```python
from build123d import *

# Parameters (mm, degrees)
SKETCH_1_W           = 20
SKETCH_1_H           = 39.9
SKETCH_1_R           = 1.5
EXTRUDE_1_DEPTH      = 5
EXTRUDE_1_2_DEPTH    = 5
EXTRUDE_2_DEPTH      = 4
EXTRUDE_2_DEPTH_BACK = 4
FILLET_1_R           = 14
SKETCH_3_R           = 1.5
CUT_EXTRUDE_1_DEPTH  = 11
FILLET_2_R           = 5
SKETCH_4_W           = 4
SKETCH_4_H           = 12
EXTRUDE_3_DEPTH      = 7
CUT_EXTRUDE_2_DEPTH  = 148
EXTRUDE_4_DEPTH      = 4
EXTRUDE_4_DEPTH_BACK = 8
SKETCH_6_W           = 4
SKETCH_6_H           = 30.5
SKETCH_10_W          = 20
SKETCH_10_H          = 6
SKETCH_10_H_2        = 5
EXTRUDE_6_DEPTH      = 4
CUT_EXTRUDE_5_DEPTH  = 6
SKETCH_13_R          = 1.5
CUT_EXTRUDE_6_DEPTH  = 6
EXTRUDE_8_DEPTH      = 4
SKETCH_19_W          = 8
SKETCH_19_H          = 15
SKETCH_19_R          = 1.5
SKETCH_19_H_2        = 8
EXTRUDE_9_DEPTH      = 5
CHAMFER_START        = -4
CHAMFER_1_DEPTH      = 8
FILLET_13_R          = 1
FILLET_14_R          = 10
FILLET_15_R          = 3


with BuildPart() as part:
    # Sketch 1 → Extrude 1 (new body)
    with BuildSketch(Plane.XY):
        with Locations((45, 0)):
            Rectangle(SKETCH_1_W, SKETCH_1_H)
        with Locations((37.5, 8)):
            Circle(SKETCH_1_R, mode=Mode.SUBTRACT)
        with Locations(Location((52.5, 8, 0), (0, 0, 180))):
            Circle(SKETCH_1_R, mode=Mode.SUBTRACT)
        with Locations((52.5, -8)):
            Circle(SKETCH_1_R, mode=Mode.SUBTRACT)
        with Locations(Location((37.5, -8, 0), (0, 0, 180))):
            Circle(SKETCH_1_R, mode=Mode.SUBTRACT)
    extrude(amount=EXTRUDE_1_DEPTH)



with BuildPart() as body_2:
    # Sketch 1 → Extrude 1 2 (new body)
    with BuildSketch(Plane.XY):
        with Locations((-45, 0)):
            Rectangle(SKETCH_1_W, SKETCH_1_H)
        with Locations((-37.5, -8)):
            Circle(SKETCH_1_R, mode=Mode.SUBTRACT)
        with Locations(Location((-52.5, -8, 0), (0, 0, 180))):
            Circle(SKETCH_1_R, mode=Mode.SUBTRACT)
        with Locations((-52.5, 8)):
            Circle(SKETCH_1_R, mode=Mode.SUBTRACT)
        with Locations(Location((-37.5, 8, 0), (0, 0, 180))):
            Circle(SKETCH_1_R, mode=Mode.SUBTRACT)
    extrude(amount=EXTRUDE_1_2_DEPTH)


with BuildPart() as part_1:
    add(part.part)

    add(body_2.part)  # Extrude 2 merges body 2
    # Sketch 2 → Extrude 2 (add, two sides: drawn at the far end of the back side and taken through both)
    with BuildSketch(Plane(origin=(0, 0, 0), x_dir=(1, 0, 0), z_dir=(0, 1, 0)).offset(-EXTRUDE_2_DEPTH_BACK)):
        Polygon((-35, -5), (-55, -5), (-30, -35), (30, -35), (55, -5), (35, -5), (35, -22), (-35, -22), align=None)
    extrude(amount=EXTRUDE_2_DEPTH + EXTRUDE_2_DEPTH_BACK)

    # Fillet 1
    fillet_1_edges = [part_1.edges().sort_by_distance(p)[0] for p in [
        (-35, 0, 22),
        (35, 0, 22),
    ]]
    fillet(fillet_1_edges, radius=FILLET_1_R)

    # Sketch 3 → Cut-Extrude 1 (cut)
    with BuildSketch(Plane(origin=(0, 4, 0), x_dir=(1, 0, 0), z_dir=(0, 1, 0))):
        with Locations(Location((17.5, -29, 0), (0, 0, 270))):
            Circle(SKETCH_3_R)
        with Locations(Location((-18.5, -29, 0), (0, 0, 270))):
            Circle(SKETCH_3_R)
        with Locations(Location((-35, -20, 0), (0, 0, 270))):
            Circle(SKETCH_3_R)
        with Locations(Location((36, -20, 0), (0, 0, 270))):
            Circle(SKETCH_3_R)
    extrude(amount=-CUT_EXTRUDE_1_DEPTH, mode=Mode.SUBTRACT)

    # Fillet 2
    fillet_2_edges = [part_1.edges().sort_by_distance(p)[0] for p in [
        (30, 0, 35),
        (-30, 0, 35),
    ]]
    fillet(fillet_2_edges, radius=FILLET_2_R)

    # Sketch 4 → Extrude 3 (add)
    with BuildSketch(Plane.XY.offset(5)):
        with Locations((-45, 10)):
            Rectangle(SKETCH_4_W, SKETCH_4_H)
        with Locations((-45, -10)):
            Rectangle(SKETCH_4_W, SKETCH_4_H)
        with Locations((45, -10)):
            Rectangle(SKETCH_4_W, SKETCH_4_H)
        with Locations((45, 10)):
            Rectangle(SKETCH_4_W, SKETCH_4_H)
    extrude(amount=EXTRUDE_3_DEPTH)

    # Sketch 5 → Cut-Extrude 2 (cut)
    with BuildSketch(Plane.ZY.offset(47)):
        Polygon((5, 16), (12, 16), (12, 4), align=None)
        Polygon((12, -16), (12, -4), (5, -16), align=None)
    extrude(amount=-CUT_EXTRUDE_2_DEPTH, mode=Mode.SUBTRACT)

    # Sketch 6 → Extrude 4 (add, two sides: drawn at the far end of the back side and taken through both)
    with BuildSketch(Plane(origin=(0, 4, 0), x_dir=(1, 0, 0), z_dir=(0, 1, 0)).offset(-EXTRUDE_4_DEPTH_BACK)):
        with Locations((11.78, -6.75)):
            Rectangle(SKETCH_6_W, SKETCH_6_H)
    extrude(amount=EXTRUDE_4_DEPTH + EXTRUDE_4_DEPTH_BACK)

    # Sketch 10 → Extrude 6 (add)
    with BuildSketch(Plane(origin=(13.78, 0, 0), x_dir=(0, 0, -1), z_dir=(1, 0, 0))):
        with Locations((-1.5, 11)):
            Rectangle(SKETCH_10_W, SKETCH_10_H)
        with Locations((-1.5, -6.5)):
            Rectangle(SKETCH_10_W, SKETCH_10_H_2)
    extrude(amount=-EXTRUDE_6_DEPTH)

    # Sketch 11 → Cut-Extrude 5 (cut)
    with BuildSketch(Plane.ZY.offset(-9.78)):
        Polygon((17.8, 8), (22, 8), (22, 4), align=None)
    extrude(amount=-CUT_EXTRUDE_5_DEPTH, mode=Mode.SUBTRACT)

    # Sketch 13 → Cut-Extrude 6 (cut)
    with BuildSketch(Plane(origin=(13.78, 0, 0), x_dir=(0, 0, -1), z_dir=(1, 0, 0))):
        with Locations((6, 9)):
            Circle(SKETCH_13_R)
        with Locations((6, -5)):
            Circle(SKETCH_13_R)
        with Locations((-9, 7)):
            Circle(SKETCH_13_R)
        with Locations((-9, -4)):
            Circle(SKETCH_13_R)
    extrude(amount=-CUT_EXTRUDE_6_DEPTH, mode=Mode.SUBTRACT)

    # Sketch 18 → Extrude 8 (add)
    with BuildSketch(Plane(origin=(13.78, 0, 0), x_dir=(0, 0, -1), z_dir=(1, 0, 0))):
        Polygon((-11.5, -9), (-11.5, -4), (-22.5, -4), align=None)
        Polygon((-17.8, 8), (-11.5, 14), (-11.5, 8), align=None)
    extrude(amount=-EXTRUDE_8_DEPTH)

    # Sketch 19 → Extrude 9 (add)
    # profile 1 of 6: a face of its own
    with BuildSketch(Plane.XY.offset(35)):
        with Locations((-19.5, 11.5)):
            Rectangle(SKETCH_19_W, SKETCH_19_H)
        with Locations((-19.5, 14.5)):
            Circle(SKETCH_19_R, mode=Mode.SUBTRACT)
    # profile 2 of 6: a face of its own
    with BuildSketch(Plane.XY.offset(35)):
        with Locations((-19.5, 0)):
            Rectangle(SKETCH_19_W, SKETCH_19_H_2)
    # profile 3 of 6: a face of its own
    with BuildSketch(Plane.XY.offset(35)):
        with Locations((-19.5, -11.5)):
            Rectangle(SKETCH_19_W, SKETCH_19_H)
        with Locations((-19.5, -14)):
            Circle(SKETCH_19_R, mode=Mode.SUBTRACT)
    # profile 4 of 6: a face of its own
    with BuildSketch(Plane.XY.offset(35)):
        with Locations((19.5, 11.5)):
            Rectangle(SKETCH_19_W, SKETCH_19_H)
        with Locations((19.5, 14)):
            Circle(SKETCH_19_R, mode=Mode.SUBTRACT)
    # profile 5 of 6: a face of its own
    with BuildSketch(Plane.XY.offset(35)):
        with Locations((19.5, 0)):
            Rectangle(SKETCH_19_W, SKETCH_19_H_2)
    # profile 6 of 6: a face of its own
    with BuildSketch(Plane.XY.offset(35)):
        with Locations((19.5, -11.5)):
            Rectangle(SKETCH_19_W, SKETCH_19_H)
        with Locations((19.5, -15.5)):
            Circle(SKETCH_19_R, mode=Mode.SUBTRACT)
    extrude(amount=EXTRUDE_9_DEPTH)

    # Chamfer 1: read off the stored shape, not the designer's step
    # Chamfer 1 outline → Chamfer 1 (add)
    with BuildSketch(Plane(origin=(0, 0, 0), x_dir=(1, 0, 0), z_dir=(0, 1, 0)).offset(CHAMFER_START)):
        with BuildLine():
            Line((23.5, -39.964499332), (28.079062635, -34.982249666))
            ThreePointArc((28.079062635, -34.982249666), (27.868780996, -34.995560446), (27.65812527, -35))
            Line((27.65812527, -35), (23.5, -35))
            Line((23.5, -35), (23.5, -39.964499332))
        make_face()
        with BuildLine():
            Line((-28.079062635, -34.982249666), (-23.5, -39.964499332))
            Line((-23.5, -39.964499332), (-23.5, -35))
            Line((-23.5, -35), (-27.65812527, -35))
            ThreePointArc((-27.65812527, -35), (-27.868780996, -34.995560446), (-28.079062635, -34.982249666))
        make_face()
        Polygon((15.5, -35), (10.5, -35), (15.5, -40), align=None)
        Polygon((-15.5, -40), (-10.5, -35), (-15.5, -35), align=None)
    extrude(amount=CHAMFER_1_DEPTH)

    # Fillet 13
    fillet_13_edges = [part_1.edges().sort_by_distance(p)[0] for p in [
        (-19.5, -19, 35),
        (-19.5, 19, 35),
        (-15.5, 19, 37.5),
        (-23.5, 19, 37.5),
        (-19.5, -19, 40),
        (-23.5, -19, 37.5),
        (-15.5, -19, 37.5),
        (-19.5, 19, 40),
        (15.5, 19, 37.5),
        (19.5, -19, 35),
        (15.5, -19, 37.5),
        (23.5, -19, 37.5),
        (19.5, 19, 40),
        (23.5, 19, 37.5),
        (19.5, -19, 40),
        (19.5, 19, 35),
    ]]
    fillet(fillet_13_edges, radius=FILLET_13_R)

    # Fillet 14
    # the kernel refuses this fillet: 10 mm, written as the material it adds along each edge
    with BuildSketch(Plane(origin=(13.78, -4, 22), x_dir=(0.9741093226814803, 0, -0.2260774811099678), z_dir=(0, 1, 0))) as fillet_14_piece_1:
        with BuildLine():
            CenterArc((12.255970323, 8.57517936), FILLET_14_R, 166.93375399, 134.02721721)
            Line((2.514877096, 10.835954171), (1.540767773, 11.062031652))
            Line((1.540767773, 11.062031652), (-0.974109323, 0.226077481))
            Line((-0.974109323, 0.226077481), (-0.226077481, -0.974109323))
            ThreePointArc((-0.226077481, -0.974109323), (6.806991829, -2.606388736), (17.914965085, -0.857517936))
            Line((17.914965085, -0.857517936), (17.400511016, 0))
        make_face()
    extrude(amount=8)
    with BuildSketch(Plane(origin=(9.78, -4, 22), x_dir=(-1, 0, 0), z_dir=(0, 1, 0))) as fillet_14_piece_2_section:
        with BuildLine():
            CenterArc((FILLET_14_R, -FILLET_14_R), FILLET_14_R, 90, 90)
            Line((0, -FILLET_14_R), (0, 0))
            Line((0, 0), (FILLET_14_R, 0))
        make_face()
    fillet_14_piece_2 = extrude(amount=8, mode=Mode.PRIVATE)
    fillet_14_piece_2 = split(fillet_14_piece_2, bisect_by=Plane(origin=(9.78, 0.195005945, 25.995243757), z_dir=(0, -0.7241379310344828, -0.6896551724137933)), keep=Keep.TOP, mode=Mode.PRIVATE)
    add(fillet_14_piece_2)
    with BuildSketch(Plane(origin=(9.78, -4, 22), x_dir=(-1, 0, 0), z_dir=(0, 1, 0))) as fillet_14_piece_3_section:
        with BuildLine():
            CenterArc((FILLET_14_R, -FILLET_14_R), FILLET_14_R, 90, 90)
            Line((0, -FILLET_14_R), (0, 0))
            Line((0, 0), (FILLET_14_R, 0))
        make_face()
    fillet_14_piece_3 = extrude(amount=33, mode=Mode.PRIVATE)
    fillet_14_piece_3 = split(fillet_14_piece_3, bisect_by=Plane(origin=(9.78, 4, 22), z_dir=(0, 1, 0)), keep=Keep.TOP, mode=Mode.PRIVATE)
    fillet_14_piece_3 = split(fillet_14_piece_3, bisect_by=Plane(origin=(9.78, 0.195005945, 25.995243757), z_dir=(0, -0.7241379310344828, -0.6896551724137933)), keep=Keep.TOP, mode=Mode.PRIVATE)
    add(fillet_14_piece_3)

    # Fillet 15
    fillet_15_edges = [part_1.edges().sort_by_distance(p)[0] for p in [
        (11.78, 14, -8.5),
        (11.78, -9, -8.5),
    ]]
    fillet(fillet_15_edges, radius=FILLET_15_R)


solid = part_1.part
```
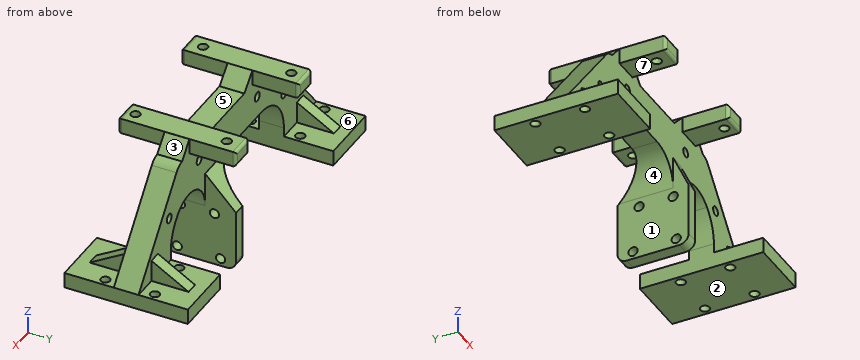
Can you work these out from the model? Positions are in its coordinate system, mm. Face numbers are marked on the shaded views. A direction names the side the tool comes from. Coordinates: 2 decimals unless noted, no trailing zeros. Order: outer loops, then holes, each group sorted by start corner. A loop starts at its lowest first (then second) coordinate and runs counter-clockwise, first axis right, second up. Notation, with made-up numbers: (46, 27.25) - (69, 27.25) arc R7 cw to (69, 40.25) - close; hole circle Ø1 at (79.25, -38.5). An arc over 180 degrees is marked (long way). Answer in a Markdown table with one row per item.
1. Suppose I cut it at B-B (x = 25.5). Please give me the cut outline in (y, z), and give its area (3 significant figures).
Reply:
| item | result |
|---|---|
| outline | (-4, 20.73) - (4, 20.73) - (4, 37.79) - (-4, 37.79) - close |
| area | 136 mm^2 |
2. For the marked faces 4, 5, 6 and 7, which set-ups out of +Z, -Z, +X, -X, +Y, -Y let a thin tool reach every point of the face, with its end or its side?
Reply:
| item | result |
|---|---|
| face 4 | -Z, +Y, -Y |
| face 5 | +Z, +Y, -Y |
| face 6 | +Z, +Y |
| face 7 | -Z, +X, -X, -Y |
3. For pin 1 (5.5 mm diameter, centred on y = -7.5, z = 9.5, fed in from -X); pin 2 (10 mm diameter, centred on y = 4, z = 16, fed in from -X); pin 3 (8 mm diameter, centred on x = -38.5, z = 10, fed in from +Y); pin 4 (6 mm diameter, centred on x = -42.5, z = 6.5, fed in from -Y), each with a flat end and sliding along its axis, tell me the tip position at first contact or that it passes through.
Reply:
| item | result |
|---|---|
| pin 1 | stops at x = -47 |
| pin 2 | stops at x = -50 |
| pin 3 | stops at y = 4 |
| pin 4 | stops at y = -19.95 |
4. If we mould it in two halves opening along X, with no side actions, what happens to the marked faces 1, 2 and 3? For each: pulls with the +X half, pulls with the -X half, needs draft (parallel to the pull), parting line crosses it, or undercut.
Reply:
| item | result |
|---|---|
| face 1 | undercut |
| face 2 | needs draft |
| face 3 | pulls with the +X half |
5. If I drill on line 1 along Y through (x, z) = (19.5, 37.4); line 2 along X through (y, z) = (-1, 29); line 3 along X through (y, z) = (1, 30), over which ranges is the centre line in solid material (lowest first)?
Reply:
| item | result |
|---|---|
| line 1 | y = -19 to -17, -14 to 12.5, 15.5 to 19 |
| line 2 | x = -35 to -20, -17 to 16, 19 to 35 |
| line 3 | x = -34.17 to -19.62, -17.38 to 16.38, 18.62 to 34.17 |
6. Suppose I cut it at A-A (x = 12.5). Please give me the cut outline in (y, z), and give its area (3 significant figures).
Reply:
| item | result |
|---|---|
| outline | (-9, -5.5) arc R3 ccw to (-6, -8.5) - (11, -8.5) arc R3 ccw to (14, -5.5) - (14, 11.5) - (4, 22) - (4, 37) - (-4, 37) - (-4, 22.5) - (-9, 11.5) - close; hole circle Ø3 at (-5, -6); hole circle Ø3 at (-4, 9); hole circle Ø3 at (7, 9); hole circle Ø3 at (9, -6) |
| area | 712 mm^2 |
